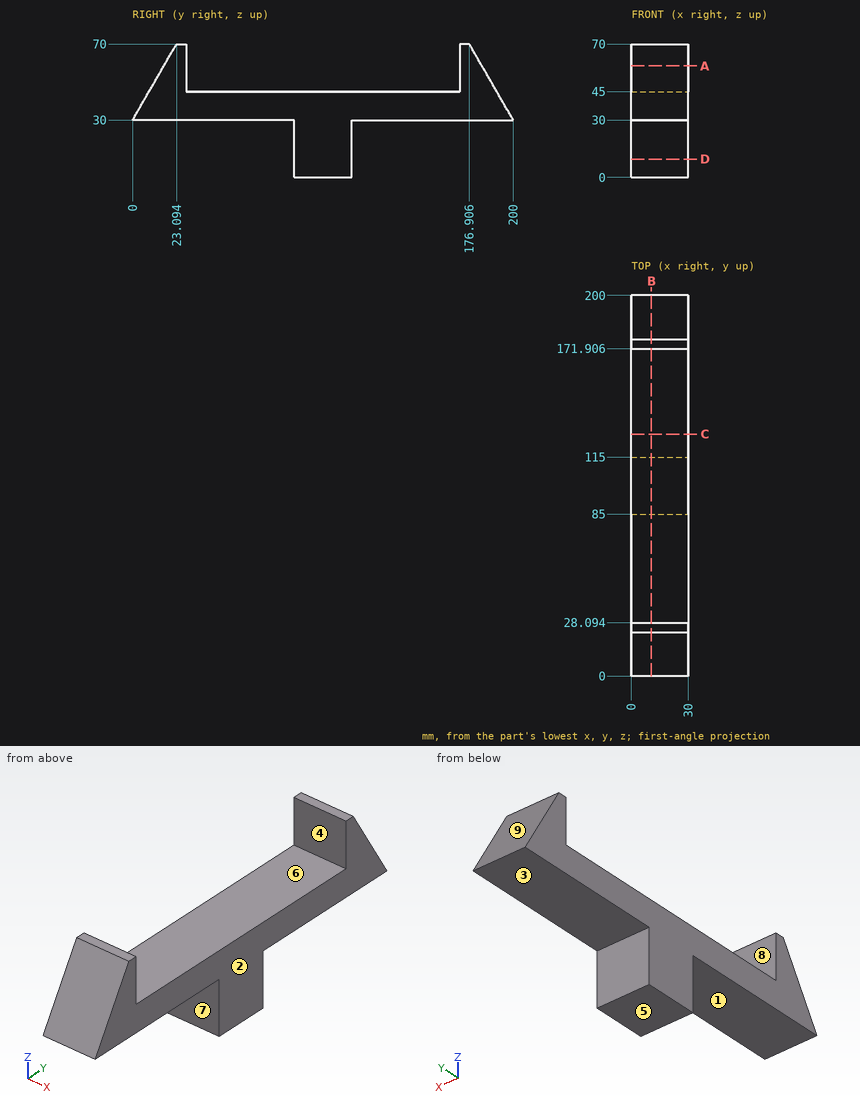
The figure shows three views and two pictorial views of one solid part (mm, origin at its lowest corner). Answer the questions. A direction names the side the tool comes from. Coordinates: 2 decimals unless noted, no trailing zeros. Loops run counter-clockwise (first coordinate to the right, second up) from the corner with the lowest first, then second, coordinate; pieces in that order, holes last. Notation, with made-up numbers: (74, 22) -> (101, 22) arc R34 cw to (101, 54) -> close; hole circle Ø7 at (73.25, 20). An arc over 180 degrees is marked (long way). Return JSON: item names as keys, results as strings. Group by question number.
(1) A cutting plane is placed at C-C on y = 127. Write down the section's boundary in (x, z).
(2) Determine the mould class of the marked faces 6, 7, 8 and 9 for opening direction Y: released by +Y, released by -Y, zero draft, split by the parting line, or undercut.
(3) Which of the six approach directions +Z, -Z, +X, -X, +Y, -Y give full straight-line access (tool end or side, diameter ignored) to the marked faces 1, 2, 3, 4 and 5?
(4) A cutting plane is placed at B-B on x = 10.5. Write down the section's boundary in (y, z).
(5) Find the intervals of material crossed by probe 1 along Z at (x, y) = (13.75, 85.5); probe 2 along Z at (x, y) = (10.5, 57.5); probe 3 along Y at (x, z) = (12.75, 15), in increasing order. Write a range as from..to.
(6) A cutting plane is placed at A-A on z = 58.5. Write down the section's boundary in (x, y).
(7) A cutting plane is placed at D-D on z = 9.5. Write down the section's boundary in (x, y).
(8) Given pin 1 Ø15 at (x, y) = (16.5, 59) entering from -Z; pin 2 Ø9 at (x, y) = (16.5, 113) entering from +Z; pin 3 Ø7.5 at (x, z) = (19, 56) entering from -Y, each flat-ended and moving along its own axis, determine where each tip first touches the part or whether it passes through.
The answers:
{
 "1": {"outline": "(0, 30) -> (30, 30) -> (30, 45) -> (0, 45) -> close"},
 "2": {"face 6": "undercut", "face 7": "released by -Y", "face 8": "undercut", "face 9": "released by +Y"},
 "3": {"face 1": "-Z, +X, -X, -Y", "face 2": "+Z, -Z, +X, +Y, -Y", "face 3": "-Z, +X, -X, +Y", "face 4": "+Z, +X, -X", "face 5": "-Z, +X, -X, +Y, -Y"},
 "4": {"outline": "(0, 30) -> (85, 30) -> (85, 0) -> (115, 0) -> (115, 30) -> (200, 30) -> (176.91, 70) -> (171.91, 70) -> (171.91, 45) -> (28.09, 45) -> (28.09, 70) -> (23.09, 70) -> close"},
 "5": {"probe 1": "z = 0..45", "probe 2": "z = 30..45", "probe 3": "y = 85..115"},
 "6": {"outline": "(0, 16.45) -> (30, 16.45) -> (30, 28.09) -> (0, 28.09) -> close; (0, 171.91) -> (30, 171.91) -> (30, 183.55) -> (0, 183.55) -> close"},
 "7": {"outline": "(0, 85) -> (30, 85) -> (30, 115) -> (0, 115) -> close"},
 "8": {"pin 1": "stops at z = 30", "pin 2": "stops at z = 45", "pin 3": "stops at y = 12.85"}
}
